```python
from build123d import *

# Parameters (mm, degrees)
F0_W     = 16.256
F0_H     = 12.954
F1_DEPTH = 16.51
F2_DEPTH = 19.05


with BuildPart() as f1:
    # F0 (on Top) → F1 (new body)
    with BuildSketch(Plane.XY):
        with BuildLine():
            Line((457.2, 141.097), (457.2, 222.25))
            Line((457.2, 222.25), (-457.2, 222.25))
            Line((-457.2, 222.25), (-457.2, 141.097))
            Line((-457.2, 141.097), (-440.357985, 141.097))
            ThreePointArc((-440.357985, 141.097), (-437.388, 133.35), (-440.357985, 125.603))
            Line((-440.357985, 125.603), (-457.2, 125.603))
            Line((-457.2, 125.603), (-457.2, -125.603))
            Line((-457.2, -125.603), (-440.357985, -125.603))
            ThreePointArc((-440.357985, -125.603), (-437.388, -133.35), (-440.357985, -141.097))
            Line((-440.357985, -141.097), (-457.2, -141.097))
            Line((-457.2, -141.097), (-457.2, -222.25))
            Line((-457.2, -222.25), (457.2, -222.25))
            Line((457.2, -222.25), (457.2, -141.097))
            Line((457.2, -141.097), (440.357985, -141.097))
            ThreePointArc((440.357985, -141.097), (437.388, -133.35), (440.357985, -125.603))
            Line((440.357985, -125.603), (457.2, -125.603))
            Line((457.2, -125.603), (457.2, 125.603))
            Line((457.2, 125.603), (440.357985, 125.603))
            ThreePointArc((440.357985, 125.603), (437.388, 133.35), (440.357985, 141.097))
            Line((440.357985, 141.097), (457.2, 141.097))
        make_face()
        with BuildLine():
            Line((457.2, 125.603), (457.2, 141.097))
            Line((457.2, 141.097), (440.357985, 141.097))
            ThreePointArc((440.357985, 141.097), (437.388, 133.35), (440.357985, 125.603))
            Line((440.357985, 125.603), (457.2, 125.603))
        make_face()
        with BuildLine():
            Line((-440.357985, 141.097), (-457.2, 141.097))
            Line((-457.2, 141.097), (-457.2, 139.827))
            Line((-457.2, 139.827), (-440.944, 139.827))
            ThreePointArc((-440.944, 139.827), (-438.658, 133.35), (-440.944, 126.873))
            Line((-440.944, 126.873), (-457.2, 126.873))
            Line((-457.2, 126.873), (-457.2, 125.603))
            Line((-457.2, 125.603), (-440.357985, 125.603))
            ThreePointArc((-440.357985, 125.603), (-437.388, 133.35), (-440.357985, 141.097))
        make_face()
        with Locations((-449.072, 133.35)):
            Rectangle(F0_W, F0_H)
        with BuildLine():
            Line((457.2, -141.097), (457.2, -125.603))
            Line((457.2, -125.603), (440.357985, -125.603))
            ThreePointArc((440.357985, -125.603), (437.388, -133.35), (440.357985, -141.097))
            Line((440.357985, -141.097), (457.2, -141.097))
        make_face()
        with BuildLine():
            Line((-440.357985, -125.603), (-457.2, -125.603))
            Line((-457.2, -125.603), (-457.2, -126.873))
            Line((-457.2, -126.873), (-440.944, -126.873))
            ThreePointArc((-440.944, -126.873), (-438.658, -133.35), (-440.944, -139.827))
            Line((-440.944, -139.827), (-457.2, -139.827))
            Line((-457.2, -139.827), (-457.2, -141.097))
            Line((-457.2, -141.097), (-440.357985, -141.097))
            ThreePointArc((-440.357985, -141.097), (-437.388, -133.35), (-440.357985, -125.603))
        make_face()
        with Locations((-449.072, -133.35)):
            Rectangle(F0_W, F0_H)
        with BuildLine():
            ThreePointArc((-440.944, 126.873), (-438.658, 133.35), (-440.944, 139.827))
            Line((-440.944, 139.827), (-440.944, 126.873))
        make_face()
        with BuildLine():
            ThreePointArc((-440.944, -139.827), (-438.658, -133.35), (-440.944, -126.873))
            Line((-440.944, -126.873), (-440.944, -139.827))
        make_face()
    extrude(amount=-F1_DEPTH)

    # F0 (on Top) → F2 (join)
    with BuildSketch(Plane.XY):
        with BuildLine():
            Line((457.2, 141.097), (457.2, 222.25))
            Line((457.2, 222.25), (-457.2, 222.25))
            Line((-457.2, 222.25), (-457.2, 141.097))
            Line((-457.2, 141.097), (-440.357985, 141.097))
            ThreePointArc((-440.357985, 141.097), (-437.388, 133.35), (-440.357985, 125.603))
            Line((-440.357985, 125.603), (-457.2, 125.603))
            Line((-457.2, 125.603), (-457.2, -125.603))
            Line((-457.2, -125.603), (-440.357985, -125.603))
            ThreePointArc((-440.357985, -125.603), (-437.388, -133.35), (-440.357985, -141.097))
            Line((-440.357985, -141.097), (-457.2, -141.097))
            Line((-457.2, -141.097), (-457.2, -222.25))
            Line((-457.2, -222.25), (457.2, -222.25))
            Line((457.2, -222.25), (457.2, -141.097))
            Line((457.2, -141.097), (440.357985, -141.097))
            ThreePointArc((440.357985, -141.097), (437.388, -133.35), (440.357985, -125.603))
            Line((440.357985, -125.603), (457.2, -125.603))
            Line((457.2, -125.603), (457.2, 125.603))
            Line((457.2, 125.603), (440.357985, 125.603))
            ThreePointArc((440.357985, 125.603), (437.388, 133.35), (440.357985, 141.097))
            Line((440.357985, 141.097), (457.2, 141.097))
        make_face()
    extrude(amount=-F2_DEPTH)


solid = f1.part
```
For this review, take the finished solid that the model builds, in its own axes (mm). A direction names the side the tool comes from. Round coordinates to 2 decimals unless told otherwise and drop trailing zeros.
(1) Tool access review of faces 4 (the flat face through (-447, -133, -16.51)), 5 (the flat face through (6, 222.25, -9)), 6 (the flat face through (447, -133, -16.51)): name each direction out of +Z, -Z, +X, -X, +Y, -Y from which nothing blocks a thin tool from reaching the whole face with its end or side.
Returned:
face 4: -Z, -X
face 5: +Z, -Z, +X, -X, +Y
face 6: -Z, +X
(2) Clearance check with a flat-ended pin moving along its axis: P1, Ø7.5, axis at x = -450, y = 131.5, coming from the -Z side. State where the tip first meets the part, or that it passes through.
Returned:
P1: stops at z = -16.51
(3) Mouldability with a two-part tool opening along Y and no side actions: class faces 1 (the flat face through (-6, -222.25, -9)), 2 (the flat face through (-6, 3, -19.05)), 3 (the flat face through (447, 133, -16.51)) as released by +Y, released by -Y, zero draft, split by the parting line, or undercut.
Returned:
face 1: released by -Y
face 2: zero draft
face 3: undercut
